Model file for the job. Use its own axes, mm. A direction names the side the tool comes from. Give positions to 0.01 mm unless a question says otherwise; leave off trailing zeros. Loops run counter-clockwise (first coordinate to the right, second up) from the corner with the lowest first, then second, coordinate; pieces in that order, holes last. Notation, with made-up numbers: M -32,-6 L -4,-6 A35 ccw -4,27 Z; hole C -28,53 d3. An arc over 180 degrees is marked long. Answer in a Markdown table with one row per item.
```python
from build123d import *

# Parameters (mm, degrees)
SKETCH1_W           = 152.4
SKETCH1_H           = 25.4
SKETCH1_R           = 3.048
BOSS_EXTRUDE1_DEPTH = 3.175
SKETCH3_W           = 12.7
SKETCH3_H           = 3.175
BOSS_EXTRUDE3_DEPTH = 3.175


with BuildPart() as part:
    # Sketch1 → Boss-Extrude1 (new body)
    with BuildSketch(Plane.XY):
        with Locations((76.2, 12.7)):
            Rectangle(SKETCH1_W, SKETCH1_H)
        with Locations((139.7, 12.7)):
            Circle(SKETCH1_R, mode=Mode.SUBTRACT)
        with Locations((33.56356, 12.7)):
            Circle(SKETCH1_R, mode=Mode.SUBTRACT)
    extrude(amount=BOSS_EXTRUDE1_DEPTH)

    # Sketch3 → Boss-Extrude3 (add)
    with BuildSketch(Plane(origin=(0, 25.4, 0), x_dir=(1, 0, 0), z_dir=(0, 1, 0))):
        with Locations((146.05, -1.5875)):
            Rectangle(SKETCH3_W, SKETCH3_H)
        with Locations((120.65, -1.5875)):
            Rectangle(SKETCH3_W, SKETCH3_H)
        with Locations((95.25, -1.5875)):
            Rectangle(SKETCH3_W, SKETCH3_H)
        with Locations((69.85, -1.5875)):
            Rectangle(SKETCH3_W, SKETCH3_H)
        with Locations((44.45, -1.5875)):
            Rectangle(SKETCH3_W, SKETCH3_H)
        with Locations((19.05, -1.5875)):
            Rectangle(SKETCH3_W, SKETCH3_H)
    extrude(amount=BOSS_EXTRUDE3_DEPTH)


solid = part.part
```
Q1. 3-axis set-ups, long thin cutter, end or side, ignore diameter. For faces 4 (the face through (6, 25.4, 2)), 5 (the face through (0, 13, 2)), 6 (the face through (139.7, 27, 2)): which of +Z, -Z, +X, -X, +Y, -Y reach the whole face in a straight line?
Reported:
| item | result |
|---|---|
| face 4 | +Z, -Z, -X, +Y |
| face 5 | +Z, -Z, -X, +Y, -Y |
| face 6 | +Z, -Z, +Y |
Q2. Drop flat-ended pins along their axis: pin 1 (1 mm diameter, centred on y = 27, z = 2, fed in from -X); pin 2 (3.5 mm diameter, centred on x = 33.56, y = 12.7, fed in from -Z); pin 3 (1 mm diameter, centred on x = 17.5, y = 5.5, fed in from -Z); pin 4 (1.6 mm diameter, centred on x = 4.5, z = 1, fed in from +Y). Give the stop position or say it passes through.
Reported:
| item | result |
|---|---|
| pin 1 | x = 12.7 |
| pin 2 | through |
| pin 3 | z = 0 |
| pin 4 | y = 25.4 |
Q3. Saw through at B-B (z = 2.5). Give the cut face in (x, y) (3 decimals), and give its area (3 significant figures).
Reported:
| item | result |
|---|---|
| outline | M 0,0 L 152.4,0 L 152.4,28.575 L 139.7,28.575 L 139.7,25.4 L 127,25.4 L 127,28.575 L 114.3,28.575 L 114.3,25.4 L 101.6,25.4 L 101.6,28.575 L 88.9,28.575 L 88.9,25.4 L 76.2,25.4 L 76.2,28.575 L 63.5,28.575 L 63.5,25.4 L 50.8,25.4 L 50.8,28.575 L 38.1,28.575 L 38.1,25.4 L 25.4,25.4 L 25.4,28.575 L 12.7,28.575 L 12.7,25.4 L 0,25.4 Z; hole C 33.564,12.7 d6.096; hole C 139.7,12.7 d6.096 |
| area | 4,050 mm² |
Q4. Mould opens along Y. For faces 1 (the face through (63.5, 27, 2)), 2 (the face through (31.317, 14.76, 1.565)), 3 (the face through (95, 28.575, 2)) say: released by +Y, released by -Y, zero draft, split by the parting line, or undercut.
Reported:
| item | result |
|---|---|
| face 1 | zero draft |
| face 2 | undercut |
| face 3 | released by +Y |
Q5. Saw through at A-A (y = 12.7). Give the cut face in (x, z) (3 decimals), and give its area (3 significant figures).
Reported:
| item | result |
|---|---|
| outline | M 0,0 L 30.516,0 L 30.516,3.175 L 0,3.175 Z; M 36.612,0 L 136.652,0 L 136.652,3.175 L 36.612,3.175 Z; M 142.748,0 L 152.4,0 L 152.4,3.175 L 142.748,3.175 Z |
| area | 445 mm² |
Q6. Probe probe 1 along X at (y, z) = (13.5, 1.2); probe 2 along Y at (x, z) = (85, 2.8). List the from-to ranges inside material, lowest first.
Reported:
| item | result |
|---|---|
| probe 1 | 0 to 30.62, 36.5 to 136.76, 142.64 to 152.4 |
| probe 2 | 0 to 25.4 |
